Work out the finished part from the listing and answer in its coordinate system (mm). A direction names the side the tool comes from. Coordinates: 2 decimals unless noted, no trailing zeros. Loops run counter-clockwise (first coordinate to the right, second up) from the corner with the lowest first, then second, coordinate; pieces in that order, holes last.
```python
from build123d import *

# Parameters (mm, degrees)
CROQUIS1_W              = 130
CROQUIS1_H              = 95
SALIENTE_EXTRUIR1_DEPTH = 5
CROQUIS2_R              = 34
SALIENTE_EXTRUIR2_DEPTH = 85
CROQUIS3_W              = 42
CROQUIS3_H              = 40
CORTAR_EXTRUIR1_DEPTH   = 30


with BuildPart() as part:
    # Croquis1 → Saliente-Extruir1 (new body)
    with BuildSketch(Plane.XY):
        Rectangle(CROQUIS1_W, CROQUIS1_H)
    extrude(amount=SALIENTE_EXTRUIR1_DEPTH)

    # Croquis2 → Saliente-Extruir2 (add)
    with BuildSketch(Plane.XY.offset(5)):
        with Locations((20, 0)):
            Circle(CROQUIS2_R)
    extrude(amount=SALIENTE_EXTRUIR2_DEPTH)

    # Croquis3 → Cortar-Extruir1 (cut)
    with BuildSketch(Plane.XY.offset(90)):
        with Locations((20, 0)):
            Rectangle(CROQUIS3_W, CROQUIS3_H)
    extrude(amount=-CORTAR_EXTRUIR1_DEPTH, mode=Mode.SUBTRACT)


solid = part.part
```
1. A cutting plane is placed at D-D, the plane x = 30. Give the vertices of the cut face in (y, z).
2. A cutting plane is placed at B-B, the plane x = -6.5. Give the vertices of the cut face in (y, z), then the cut area to 3 significant figures.
3. A cutting plane is placed at A-A, the plane y = 0. Give the vertices of the cut face in (x, z), then the cut area to 3 significant figures.
4. Determine the mould class of faces 3 (the flat face through (20, -22, 90)), 4 (the flat face through (41, 0, 75)), 5 (the cylindrical face through (15.57, 33.71, 46.9)) for opening direction Y: released by +Y, released by -Y, zero draft, split by the parting line, or undercut.
5. Straight lines are drawn through the part: probe 1 along Z at (x, y) = (-32, 18.5); probe 2 along Z at (x, y) = (33, -7); probe 3 along X at (y, z) = (13, 70). For each, find the intervals that lie inside material, in ascending order.
6. For faces 1 (the flat face through (65, -1, 2)), 2 (the flat face through (20, 20, 75)), determine the directions among +Z, -Z, +X, -X, +Y, -Y from which every point of the face is accessible in a straight line to the end or side of a thin tool.
7. A cutting plane is placed at C-C, the plane z = 20. Give the vertices of the cut face in (x, y), then the cut area to 3 significant figures.
8. Each of these flat-tipped pins is pushed along its axis until it touches: P1, Ø24, axis at x = 15, z = 76.5, coming from the +Y side; P2, Ø2, axis at x = -5, z = 69, coming from the +Y side; P3, Ø10, axis at y = -18.5, z = 46, coming from the -X side. Where does it stop, or does it pass through?
Answers below:
1. outline: (-47.5, 0) - (47.5, 0) - (47.5, 5) - (32.5, 5) - (32.5, 90) - (20, 90) - (20, 60) - (-20, 60) - (-20, 90) - (-32.5, 90) - (-32.5, 5) - (-47.5, 5) - close
2. outline: (-47.5, 0) - (47.5, 0) - (47.5, 5) - (21.3, 5) - (21.3, 90) - (-21.3, 90) - (-21.3, 5) - (-47.5, 5) - close
2. area: 4,100 mm2
3. outline: (-65, 0) - (65, 0) - (65, 5) - (54, 5) - (54, 90) - (41, 90) - (41, 60) - (-1, 60) - (-1, 90) - (-14, 90) - (-14, 5) - (-65, 5) - close
3. area: 5,170 mm2
4. face 3: zero draft
4. face 4: undercut
4. face 5: split by the parting line
5. probe 1: z = 0 to 5
5. probe 2: z = 0 to 60
5. probe 3: x = -11.42 to -1, 41 to 51.42
6. face 1: +Z, -Z, +X, +Y, -Y
6. face 2: +Z
7. outline: circle Ø68 at (20, 0)
7. area: 3,630 mm2
8. P1: stops at y = 34
8. P2: stops at y = 24.08
8. P3: stops at x = -11.2
